from build123d import *

# Parameters (mm, degrees)
SKETCH_1_R          = 4.1
EXTRUDE_1_DEPTH     = 20
SKETCH_2_R          = 4.923200542
EXTRUDE_2_DEPTH     = 3
CUT_EXTRUDE_1_DEPTH = 13
SKETCH_6_R          = 3.5
EXTRUDE_3_DEPTH     = 3


with BuildPart() as part:
    # Эскиз1 → Бобышка-Вытянуть1 (new body)
    with BuildSketch(Plane.XY):
        with BuildLine():
            Line((5.123475383, -4), (32.5, -4))
            Line((32.5, -4), (32.5, 0))
            Line((32.5, 0), (6.5, 0))
            ThreePointArc((6.5, 0), (-6.146242348, 2.115113473), (5.123475383, -4))
        make_face()
        Circle(SKETCH_1_R, mode=Mode.SUBTRACT)
    extrude(amount=EXTRUDE_1_DEPTH)

    # Эскиз2 → Бобышка-Вытянуть2 (add)
    with BuildSketch(Plane.XY.offset(20)):
        Circle(SKETCH_2_R)
    extrude(amount=-EXTRUDE_2_DEPTH)

    # Эскиз3 → Вырез-Вытянуть1 (cut)
    with BuildSketch(Plane(origin=(0, 0, 0), x_dir=(1, 0, 0), z_dir=(0, 1, 0))):
        with BuildLine():
            Line((10, -7.25), (13, -7.25))
            ThreePointArc((13, -7.25), (15.25, -5), (13, -2.75))
            Line((13, -2.75), (10, -2.75))
            ThreePointArc((10, -2.75), (7.75, -5), (10, -7.25))
        make_face()
        with BuildLine():
            Line((26, -2.75), (29, -2.75))
            ThreePointArc((29, -2.75), (31.25, -5), (29, -7.25))
            Line((29, -7.25), (26, -7.25))
            ThreePointArc((26, -7.25), (23.75, -5), (26, -2.75))
        make_face()
    extrude(amount=-CUT_EXTRUDE_1_DEPTH, mode=Mode.SUBTRACT)

    # Эскиз6 → Бобышка-Вытянуть3 (add)
    with BuildSketch(Plane(origin=(22.2, 0, 0), x_dir=(0, 0, -1), z_dir=(1, 0, 0))):
        with BuildLine():
            Line((-31.59202383, -22.918584172), (-20, 0))
            Line((-20, 0), (-10, -4))
            Line((-10, -4), (-18.755733241, -28.438927439))
            ThreePointArc((-18.755733241, -28.438927439), (-28.111077184, -32.508536772), (-31.59202383, -22.918584172))
        make_face()
        with Locations((-25.34557078, -26.077986693)):
            Circle(SKETCH_6_R, mode=Mode.SUBTRACT)
    extrude_3 = extrude(amount=EXTRUDE_3_DEPTH)

    # Зеркальное отражение1: Бобышка-Вытянуть3 across plane
    add(extrude_3.mirror(Plane(origin=(20, 0, 0), x_dir=(0, 0, 1), z_dir=(1, 0, 0))))


solid = part.part
For this review, take the finished solid that the model builds, in its own axes (mm). A direction names the side the tool comes from. Coordinates: 2 decimals unless noted, no trailing zeros. Order: outer loops, then holes, each group sorted by start corner. A loop starts at its lowest first (then second) coordinate and runs counter-clockwise, first axis right, second up. Notation, with made-up numbers: (81, -3.5) - (133, -3.5) arc R29 cw to (133, 30.5) - close; hole circle Ø2 at (58.25, 37). An arc over 180 degrees is marked (long way). Use one line per item in the form item = value.
Q1. Consider section B-B (z = 27.5). Give the boundary of the cut face in (x, y), then the cut area to 3 significant figures.
Checked values:
outline = (14.8, -32.74) - (17.8, -32.74) - (17.8, -28.84) - (14.8, -28.84) - close; (14.8, -23.32) - (17.8, -23.32) - (17.8, -14.83) - (14.8, -14.83) - close; (22.2, -32.74) - (25.2, -32.74) - (25.2, -28.84) - (22.2, -28.84) - close; (22.2, -23.32) - (25.2, -23.32) - (25.2, -14.83) - (22.2, -14.83) - close
area = 74.4 mm2
Q2. For faces 1 (the flat face through (19, -4, 10)), 2 (the cylindrical face through (31.25, -1.97, 4.95)), 3 (the flat face through (20, -2, 20)), 4 (the flat face through (29, -2, 20)), list the 3-axis set-ups (+Z, -Z, +X, -X, +Y, -Y) from which the entire face can be reached by the end or side of a thin tool; tool diameter is ignored.
Checked values:
face_1 = -Z, -Y
face_2 = +Y, -Y
face_3 = +Z, +Y, -Y
face_4 = +Z, +X, +Y, -Y
Q3. Draft analysis for pull direction Y (two halves, no side actions). For faces 5 (the flat face through (0, 0, 17)), 6 (the flat face through (27, -2, 2.75)), 7 (the flat face through (16.3, -16, 14.3)), 8 (the cylindrical face through (16.32, -28.21, 28.12)), state which applies: +Y half, -Y half, draft (parallel to the pull), parting line (faces both ways), or undercut.
Checked values:
face_5 = undercut
face_6 = draft
face_7 = -Y half
face_8 = undercut
Q4. For P1, Ø6.5, axis at x = 0, y = 0, coming from the +Z side; P2, Ø18, axis at y = -21.5, z = 26.5, coming from the +X side; P3, Ø10, axis at x = 21.5, y = -19, coming from the +Z side, all flat-tipped, find the tip position at first contact; note any pin that passes through.
Checked values:
P1 = 20
P2 = 25.2
P3 = 32.01
Q5. Consider section A-A (z = 5). Give the boundary of the cut face in (x, y), then the cut area to 3 significant figures.
Checked values:
outline = (5.12, -4) - (7.75, -4) - (7.75, 0) - (6.5, 0) arc R6.5 ccw (long way) to start; (15.25, -4) - (23.75, -4) - (23.75, 0) - (15.25, 0) - close; (31.25, -4) - (32.5, -4) - (32.5, 0) - (31.25, 0) - close; hole circle Ø8.2 at (0, 0)
area = 126 mm2
Q6. Consider section C-C (y = -16). Give the boundary of the cut face in (x, z).
Checked values:
outline = (14.8, 14.3) - (17.8, 14.3) - (17.8, 28.09) - (14.8, 28.09) - close; (22.2, 14.3) - (25.2, 14.3) - (25.2, 28.09) - (22.2, 28.09) - close
Q7. Consider section D-D (x = 30.5). Give the boundary of the cut face in (y, z), then the cut area to 3 significant figures.
Checked values:
outline = (-4, 0) - (0, 0) - (0, 3.32) - (-4, 3.32) - close; (-4, 6.68) - (0, 6.68) - (0, 20) - (-4, 20) - close
area = 66.6 mm2
Q8. For probe 1 along Z at (x, y) = (28.5, -3.5); probe 2 along X at (y, z) = (-16, 22.5); probe 3 along Y at (x, z) = (0, 6.25), list the stretches that pass through material, from the lowest coordinate up. Write a range as from..to.
Checked values:
probe_1 = 0..2.75, 7.25..20
probe_2 = 14.8..17.8, 22.2..25.2
probe_3 = -6.5..-4.1, 4.1..6.5
